Verification items for the finished model (mm, model axes). Round coordinates to 2 decimals unless told otherwise and drop trailing zeros. Loops run counter-clockwise (first coordinate to the right, second up) from the corner with the lowest first, then second, coordinate; pieces in that order, holes last. Notation, with made-up numbers: M 30,6.5 L 75,6.5 A7 ccw 75,12.5 Z; hole C 87,78.5 d7. An arc over 180 degrees is marked long. Write item = value, one per line. Start each with the question number.
from build123d import *

# Parameters (mm, degrees)
SKETCH1_W           = 50
SKETCH1_H           = 50
BOSS_EXTRUDE1_DEPTH = 10
FILLET1_R           = 2
FILLET2_R           = 2
FILLET3_R           = 2
FILLET4_R           = 2
FILLET5_R           = 2


with BuildPart() as part:
    # Sketch1 → Boss-Extrude1 (new body)
    with BuildSketch(Plane(origin=(0, 0, 0), x_dir=(1, 0, 0), z_dir=(0, 1, 0))):
        Rectangle(SKETCH1_W, SKETCH1_H)
    extrude(amount=BOSS_EXTRUDE1_DEPTH)

    # Fillet1
    fillet1_edges = [part.edges().sort_by_distance(p)[0] for p in [
        (0, 10, 25),
    ]]
    fillet(fillet1_edges, radius=FILLET1_R)

    # Fillet2
    fillet2_edges = [part.edges().sort_by_distance(p)[0] for p in [
        (25, 10, -1),
        (25, 4, 25),
        (25, 9.414213562, 24.414213562),
    ]]
    fillet(fillet2_edges, radius=FILLET2_R)

    # Fillet3
    fillet3_edges = [part.edges().sort_by_distance(p)[0] for p in [
        (25, 4, -25),
        (-1, 10, -25),
        (24.414213562, 9.414213562, -25),
    ]]
    fillet(fillet3_edges, radius=FILLET3_R)

    # Fillet4
    fillet4_edges = [part.edges().sort_by_distance(p)[0] for p in [
        (-25, 4, 25),
        (-25, 9.414213562, 24.414213562),
        (-25, 4, -25),
        (-25, 10, 0),
        (-25, 9.414213562, -24.414213562),
    ]]
    fillet(fillet4_edges, radius=FILLET4_R)

    # Fillet5
    fillet5_edges = [part.edges().sort_by_distance(p)[0] for p in [
        (25, 0, 0),
        (24.414213562, 0, 24.414213562),
        (0, 0, -25),
        (24.414213562, 0, -24.414213562),
        (-25, 0, 0),
        (0, 0, 25),
        (-24.414213562, 0, 24.414213562),
        (-24.414213562, 0, -24.414213562),
    ]]
    fillet(fillet5_edges, radius=FILLET5_R)


solid = part.part
1. Section check A-A, the plane y = 9.25. Enter the section's corners in (x, z), and give its area (3 significant figures).
2. Gauge pin test, flat end, axial feed: P1, Ø4, axis at x = 3, y = 9, coming from the +Z side. Record the tip position at first contact, or that the pin passes through.
3. Thickness scan on line 1 (Z direction, x = 12, y = 1.25); line 2 (Z direction, x = -13.5, y = 1.75); line 3 (X direction, y = 1, z = 8.5). Record the ranges inside material, lowest first.
Computed values:
q1.outline = M -24.56,-23 A1.56 ccw -23,-24.56 L 23,-24.56 A1.56 ccw 24.56,-23 L 24.56,23 A1.56 ccw 23,24.56 L -23,24.56 A1.56 ccw -24.56,23 Z
q1.area = 2,410 mm2
q2.P1 = 25
q3.line_1 = -24.85 to 24.85
q3.line_2 = -24.98 to 24.98
q3.line_3 = -24.73 to 24.73
